Part model, mm, in its own coordinate system. Coordinates: 2 decimals unless noted, no trailing zeros. Order: outer loops, then holes, each group sorted by start corner. A loop starts at its lowest first (then second) coordinate and runs counter-clockwise, first axis right, second up.
1) Pin check, flat tips, straight feed: pin 1 Ø6 at (x, z) = (84.29, 69.6) entering from +Y; pin 2 Ø0.6 at (x, y) = (131, 0.5) entering from -Z. Stop position of each tip, or through.
2) Wall check: L1, parallel to Z at x = 84.5, y = 1.3; L2, parallel to X at y = 0.65, z = 70; L3, parallel to Z at x = 85, y = 1.8. Give the ranges that are in metal, low to high.
3) Cut at A-A (y = 1.1). List the corners of the cut face in (x, z) (3 decimals), and give its area (3 significant figures).
4) Cut at B-B (x = 114). List the corners of the cut face in (y, z).
5) Cut at C-C (z = 17.5). List the corners of the cut face in (x, y), and give its area (3 significant figures).
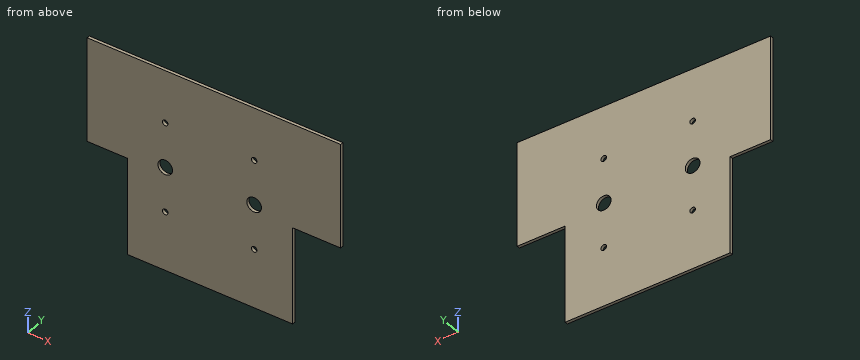
```python
from build123d import *

# Parameters (mm, degrees)
AUFSATZ_LINEAR_AUSTRAGEN1_DEPTH = 2
SKIZZE2_R                       = 4.875
SCHNITT_LINEAR_AUSTRAGEN1_DEPTH = 2
SKIZZE3_R                       = 4.875
SCHNITT_LINEAR_AUSTRAGEN2_DEPTH = 2
SKIZZE4_R                       = 1.875
SCHNITT_LINEAR_AUSTRAGEN3_DEPTH = 2
SKIZZE5_R                       = 1.845307759
SCHNITT_LINEAR_AUSTRAGEN4_DEPTH = 2
SKIZZE6_R                       = 1.875
SCHNITT_LINEAR_AUSTRAGEN5_DEPTH = 2
SKIZZE7_R                       = 1.875
SCHNITT_LINEAR_AUSTRAGEN6_DEPTH = 2


with BuildPart() as part:
    # Skizze1 → Aufsatz-Linear austragen1 (new body)
    with BuildSketch(Plane(origin=(0, 0, 0), x_dir=(1, 0, 0), z_dir=(0, 1, 0))):
        Polygon((142, -65), (110, -65), (110, 0), (0, 0), (0, -65), (-27, -65), (-27, -135), (142, -135), align=None)
    extrude(amount=AUFSATZ_LINEAR_AUSTRAGEN1_DEPTH)

    # Skizze2 → Schnitt-Linear austragen1 (cut)
    with BuildSketch(Plane(origin=(0, 2, 0), x_dir=(1, 0, 0), z_dir=(0, 1, 0))):
        with Locations((25.044083651, -69.597933498)):
            Circle(SKIZZE2_R)
    extrude(amount=-SCHNITT_LINEAR_AUSTRAGEN1_DEPTH, mode=Mode.SUBTRACT)

    # Skizze3 → Schnitt-Linear austragen2 (cut)
    with BuildSketch(Plane(origin=(0, 2, 0), x_dir=(1, 0, 0), z_dir=(0, 1, 0))):
        with Locations((84.294083651, -69.597933498)):
            Circle(SKIZZE3_R)
    extrude(amount=-SCHNITT_LINEAR_AUSTRAGEN2_DEPTH, mode=Mode.SUBTRACT)

    # Skizze4 → Schnitt-Linear austragen3 (cut)
    with BuildSketch(Plane(origin=(0, 2, 0), x_dir=(1, 0, 0), z_dir=(0, 1, 0))):
        with Locations((84.294083651, -99.672933498)):
            Circle(SKIZZE4_R)
    extrude(amount=-SCHNITT_LINEAR_AUSTRAGEN3_DEPTH, mode=Mode.SUBTRACT)

    # Skizze5 → Schnitt-Linear austragen4 (cut)
    with BuildSketch(Plane(origin=(0, 2, 0), x_dir=(1, 0, 0), z_dir=(0, 1, 0))):
        with Locations((25.044083651, -99.672933498)):
            Circle(SKIZZE5_R)
    extrude(amount=-SCHNITT_LINEAR_AUSTRAGEN4_DEPTH, mode=Mode.SUBTRACT)

    # Skizze6 → Schnitt-Linear austragen5 (cut)
    with BuildSketch(Plane(origin=(0, 2, 0), x_dir=(1, 0, 0), z_dir=(0, 1, 0))):
        with Locations((84.294083651, -39.522933498)):
            Circle(SKIZZE6_R)
    extrude(amount=-SCHNITT_LINEAR_AUSTRAGEN5_DEPTH, mode=Mode.SUBTRACT)

    # Skizze7 → Schnitt-Linear austragen6 (cut)
    with BuildSketch(Plane(origin=(0, 2, 0), x_dir=(1, 0, 0), z_dir=(0, 1, 0))):
        with Locations((25.044083651, -39.522933498)):
            Circle(SKIZZE7_R)
    extrude(amount=-SCHNITT_LINEAR_AUSTRAGEN6_DEPTH, mode=Mode.SUBTRACT)


solid = part.part
```
Geometry check:
1. pin 1: passes through
1. pin 2: stops at z = 65
2. L1: z = 0 to 37.66, 41.39 to 64.73, 74.47 to 97.81, 101.54 to 135
2. L2: x = -27 to 20.19, 29.9 to 79.44, 89.15 to 142
2. L3: z = 0 to 37.79, 41.26 to 64.77, 74.42 to 97.94, 101.41 to 135
3. outline: (-27, 65) - (0, 65) - (0, 0) - (110, 0) - (110, 65) - (142, 65) - (142, 135) - (-27, 135) - close; hole circle Ø9.75 at (25.044, 69.598); hole circle Ø3.75 at (25.044, 39.523); hole circle Ø3.691 at (25.044, 99.673); hole circle Ø9.75 at (84.294, 69.598); hole circle Ø3.75 at (84.294, 39.523); hole circle Ø3.75 at (84.294, 99.673)
3. area: 18,800 mm2
4. outline: (0, 65) - (2, 65) - (2, 135) - (0, 135) - close
5. outline: (0, 0) - (110, 0) - (110, 2) - (0, 2) - close
5. area: 220 mm2
